```python
from build123d import *

# Parameters (mm, degrees)
BOSS_EXTRUDE2_DEPTH = 15
FILLET2_R           = 2.5
SKETCH3_R           = 0.5
BOSS_EXTRUDE4_DEPTH = 2.5


with BuildPart() as part:
    # Sketch1 → Boss-Extrude2 (new body)
    with BuildSketch(Plane(origin=(0, 0, 0), x_dir=(1, 0, 0), z_dir=(0, 1, 0))):
        with BuildLine():
            Line((-23.383883476, 16.616116524), (21.616116524, 16.616116524))
            ThreePointArc((21.616116524, 16.616116524), (23.383883476, 15.883883476), (24.116116524, 14.116116524))
            Line((24.116116524, 14.116116524), (24.116116524, -15.883883476))
            ThreePointArc((24.116116524, -15.883883476), (23.383883476, -17.651650429), (21.616116524, -18.383883476))
            Line((21.616116524, -18.383883476), (-23.383883476, -18.383883476))
            ThreePointArc((-23.383883476, -18.383883476), (-25.151650429, -17.651650429), (-25.883883476, -15.883883476))
            Line((-25.883883476, -15.883883476), (-25.883883476, 14.116116524))
            ThreePointArc((-25.883883476, 14.116116524), (-25.151650429, 15.883883476), (-23.383883476, 16.616116524))
        make_face()
    extrude(amount=BOSS_EXTRUDE2_DEPTH)

    # Fillet2
    fillet2_edges = [part.edges().sort_by_distance(p)[0] for p in [
        (-25.151650429, 15, 17.651650429),
        (-25.883883476, 0, 0.883883476),
        (-25.151650429, 0, -15.883883476),
        (-0.883883476, 15, 18.383883476),
        (23.383883476, 15, 17.651650429),
        (24.116116524, 15, 0.883883476),
        (23.383883476, 15, -15.883883476),
        (-0.883883476, 15, -16.616116524),
        (-25.151650429, 15, -15.883883476),
        (-25.883883476, 15, 0.883883476),
        (-0.883883476, 0, -16.616116524),
        (23.383883476, 0, -15.883883476),
        (24.116116524, 0, 0.883883476),
        (23.383883476, 0, 17.651650429),
        (-0.883883476, 0, 18.383883476),
        (-25.151650429, 0, 17.651650429),
    ]]
    fillet(fillet2_edges, radius=FILLET2_R)

    # Sketch3 → Boss-Extrude4 (add)
    with BuildSketch(Plane(origin=(0, 0, 0), x_dir=(1, 0, 0), z_dir=(0, 1, 0))):
        with BuildLine():
            Line((-25.883883476, 16.646945133), (24.116116524, 16.646945133))
            ThreePointArc((24.116116524, 16.646945133), (29.061870418, 13.334132498), (32.766116524, 8.674328862))
            Line((32.766116524, 8.674328862), (32.766116524, -10.453501419))
            ThreePointArc((32.766116524, -10.453501419), (29.124788001, -15.055056138), (24.271254893, -18.353054867))
            Line((24.271254893, -18.353054867), (-26.039021846, -18.353054867))
            ThreePointArc((-26.039021846, -18.353054867), (-30.892554954, -15.055056138), (-34.533883476, -10.453501419))
            Line((-34.533883476, -10.453501419), (-34.533883476, 8.674328862))
            ThreePointArc((-34.533883476, 8.674328862), (-30.829637371, 13.334132498), (-25.883883476, 16.646945133))
        make_face()
        with Locations(Location((-28.883883476, 10.158483361, 0), (0, 0, 270))):
            Circle(SKETCH3_R, mode=Mode.SUBTRACT)
        with Locations(Location((-29.383883476, -11.841516639, 0), (0, 0, 270))):
            Circle(SKETCH3_R, mode=Mode.SUBTRACT)
        with Locations(Location((27.616116524, -11.841516639, 0), (0, 0, 270))):
            Circle(SKETCH3_R, mode=Mode.SUBTRACT)
        with Locations(Location((27.116116524, 10.158483361, 0), (0, 0, 270))):
            Circle(SKETCH3_R, mode=Mode.SUBTRACT)
        with BuildLine():
            Line((29.616116524, 6.658483361), (29.616116524, -8.426250314))
            ThreePointArc((29.616116524, -8.426250314), (27.616116524, -10.426250314), (25.616116524, -8.426250314))
            Line((25.616116524, -8.426250314), (25.616116524, 6.658483361))
            ThreePointArc((25.616116524, 6.658483361), (27.616116524, 8.658483361), (29.616116524, 6.658483361))
        make_face(mode=Mode.SUBTRACT)
        with BuildLine():
            Line((-31.383883476, 6.658483361), (-31.383883476, -8.426250314))
            ThreePointArc((-31.383883476, -8.426250314), (-29.383883476, -10.426250314), (-27.383883476, -8.426250314))
            Line((-27.383883476, -8.426250314), (-27.383883476, 6.658483361))
            ThreePointArc((-27.383883476, 6.658483361), (-29.383883476, 8.658483361), (-31.383883476, 6.658483361))
        make_face(mode=Mode.SUBTRACT)
    extrude(amount=BOSS_EXTRUDE4_DEPTH)


solid = part.part
```
Model file for the job. Use its own axes, mm. A direction names the side the tool comes from. Coordinates: 2 decimals unless noted, no trailing zeros. Loops run counter-clockwise (first coordinate to the right, second up) from the corner with the lowest first, then second, coordinate; pieces in that order, holes last. Notation, with made-up numbers: M 30.5,66.5 L 75.5,66.5 A22 ccw 75.5,77.5 Z; hole C 7.25,62 d9. An arc over 180 degrees is marked long. Use CSV: the item, a comma, the result in double quotes. Start each with the question number.
1. Probe probe 1 along Z at (x, y) = (-21, 5.5); probe 2 along X at (y, z) = (9.25, 0); probe 3 along Y at (x, z) = (25.5, -12.5). List the from-to ranges inside material, lowest first. Write a range as [from, to].
2. Tool access for faces 4 (the flat face through (-25.884, 7, 1)), 5 (the flat face through (25.616, 1, 1)), 6 (the cylindrical face through (-25.1, 7.4, 17.7)): list every direction of +Z, -Z, +X, -X, +Y, -Y with a clear straight run to the whole face (end or side of a thin tool).
3. Band-saw the part on C-C, the plane z = 15. List the corners of the cut face in (x, y).
4. Band-saw the part on B-B, the plane y = 3.5. List the corners of the cut face in (x, z), then the cut area to 3 significant figures.
5. Flat gauge pins, fed straight in: pin 1 (1 mm diameter, centred on x = 16, y = 8, fed in from -Z); pin 2 (2 mm diameter, centred on x = -16.5, y = 13, fed in from +Z); pin 3 (2 mm diameter, centred on y = 12.5, z = -10.5, fed in from +X); pin 4 (2 mm diameter, centred on x = -27, z = -1.5, fed in from +Y). Where does each tip first touch, or does it go through?
6. Two-plate mould, pull along X, no slides. Class faces 1 (the flat face through (32.766, 1, 1)), 2 (the cylindrical face through (27.572, 1.232, -8.658)), 3 (the flat face through (0, 0, 1)): pulls with the +X half, pulls with the -X half, needs draft (parallel to the pull), parting line crosses it, or undercut.
7. Band-saw the part on D-D, the plane z = -8. List the corners of the cut face in (x, y).
8. Band-saw the part on A-A, the plane z = 6. List the corners of the cut face in (x, y).
Entries:
1,probe 1,"z = [-16.62, 18.38]"
1,probe 2,"x = [-25.88, 24.12]"
1,probe 3,"y = [0, 2.5]"
2,face 4,"+Z, -Z, -X, +Y"
2,face 5,"+Y, -Y"
2,face 6,"+Z, -X, +Y"
3,outline,"M -30.95,0 L 29.18,0 L 29.18,2.5 L 24.12,2.5 L 24.12,12.5 A2.5 ccw 21.62,15 L -23.38,15 A2.5 ccw -25.88,12.5 L -25.88,2.5 L -30.95,2.5 Z"
4,outline,"M -25.88,-14.12 A2.5 ccw -23.38,-16.62 L 21.62,-16.62 A2.5 ccw 24.12,-14.12 L 24.12,15.88 A2.5 ccw 21.62,18.38 L -23.38,18.38 A2.5 ccw -25.88,15.88 Z"
4,area,"1,740 mm2"
5,pin 1,"stops at z = -16.62"
5,pin 2,"stops at z = 18.38"
5,pin 3,"stops at x = 24.12"
5,pin 4,"stops at y = 2.5"
6,face 1,"pulls with the +X half"
6,face 2,"undercut"
6,face 3,"needs draft"
7,outline,"M -34.53,0 L -30.87,0 L -30.87,2.5 L -34.53,2.5 Z; M -27.9,0 L 26.13,0 L 26.13,2.5 L 24.12,2.5 L 24.12,12.5 A2.5 ccw 21.62,15 L -23.38,15 A2.5 ccw -25.88,12.5 L -25.88,2.5 L -27.9,2.5 Z; M 29.1,0 L 32.77,0 L 32.77,2.5 L 29.1,2.5 Z"
8,outline,"M -34.53,0 L -31.38,0 L -31.38,2.5 L -34.53,2.5 Z; M -27.38,0 L 25.62,0 L 25.62,2.5 L 24.12,2.5 L 24.12,12.5 A2.5 ccw 21.62,15 L -23.38,15 A2.5 ccw -25.88,12.5 L -25.88,2.5 L -27.38,2.5 Z; M 29.62,0 L 32.77,0 L 32.77,2.5 L 29.62,2.5 Z"
